Can you work these out from the model? Positions are in its coordinate system, mm. A direction names the side the tool comes from. Coordinates: 2 decimals unless noted, no trailing zeros. Write each loop counter-clockwise with the first axis right and the second up, starting at its lowest first coordinate (ties: lowest second). Pieces come first, ordered by that corner, then holes. Notation, with made-up numbers: (-13, 87.5) - (-6, 87.5) arc R30 cw to (-6, 121.5) - close; hole circle Ø1 at (51.5, 73.5). An arc over 180 degrees is marked (long way). Use one line per item in the form item = value. Start each with the question number.
(1) If I drill on probe 1 along X at (y, z) = (1.7, 10); probe 2 along Z at (x, y) = (-17.5, 3); probe 3 along Z at (x, y) = (17.5, 1.85), over which ranges is the centre line in solid material (lowest first)? Write a range as from..to.
(2) If we section it at C-C on y = 3.1: Please give me the cut outline in (x, z).
(3) On a 3-axis mill with a long thin cutter (end or side, diameter ignored), from which of +Z, -Z, +X, -X, +Y, -Y can I reach the whole of each face in a straight line? I mean faces 1 (the face through (-50, 2, -9)), 2 (the face through (-25, 2, 2)). Say none if no direction works.
(4) Thinking about a two-plate mould opening in Z: for faces 3 (the face through (-18.51, 2.53, -11.11)), 4 (the face through (-1, 5, -4)), 5 (the face through (1, 2, -17.5)), which applies, pulls with the +Z half, pulls with the -Z half, needs draft (parallel to the pull), parting line crosses it, or undercut?
(5) If we section it at B-B on x = -7: Please give me the cut outline in (y, z).
(6) For pin 1 Ø2.5 at (x, z) = (17.5, 10) entering from +Y, with a flat end and sliding along its axis, tell me the tip position at first contact or that it passes through.
(7) If we section it at D-D on x = -17.5: Give the number of separate pieces and of enclosed holes in the cut face, then the cut area to 3 significant figures.
(8) If we section it at A-A on z = 10: Please give me the cut outline in (x, y), then the cut area to 3 significant figures.
```python
from build123d import *

# Parameters (mm, degrees)
BOSS_EXTRUDE1_DEPTH            = 5
F_3_0MM_DOWEL_HOLE1_AT_2_COUNT = 2
F_3_0MM_DOWEL_HOLE1_AT_2_PITCH = 40.311288741
M5_CLEARANCE_HOLE1_AT_2_COUNT  = 2
M5_CLEARANCE_HOLE1_AT_2_PITCH  = 40.311288741
CHAMFER1_SIZE                  = 1
CHAMFER2_SIZE                  = 0.2


with BuildPart() as part:
    # Sketch2 → Boss-Extrude1 (new body)
    with BuildSketch(Plane(origin=(0, 0, 0), x_dir=(1, 0, 0), z_dir=(0, 1, 0))):
        with BuildLine():
            Line((-50, 2), (0, 2))
            ThreePointArc((0, 2), (2, 0), (0, -2))
            Line((0, -2), (-50, -2))
            Line((-50, -2), (-50, -17.5))
            Line((-50, -17.5), (50, -17.5))
            Line((50, -17.5), (50, 17.5))
            Line((50, 17.5), (-50, 17.5))
            Line((-50, 17.5), (-50, 2))
        make_face()
    extrude(amount=BOSS_EXTRUDE1_DEPTH)

    # Sketch4 → Ø3.0mm Dowel Hole1 (revolve, cut)
    with BuildSketch(Plane(origin=(-17.5, 5, -10), x_dir=(0, 0, 1), z_dir=(1, 0, 0))):
        Polygon((0, 0), (0, 5), (1.75, 5), (1.5, 4.75), (1.5, 0.25), (1.75, 0), align=None)
    f_3_0mm_dowel_hole1 = revolve(axis=Axis((-17.5, 11.35, -10), (0, -1, 0)), mode=Mode.SUBTRACT)

    # Ø3.0mm Dowel Hole1 at 2: Ø3.0mm Dowel Hole1 ×2
    with Locations(*[Vector(0.8682431421244593, 0, 0.4961389383568337) * (i * F_3_0MM_DOWEL_HOLE1_AT_2_PITCH) for i in range(1, F_3_0MM_DOWEL_HOLE1_AT_2_COUNT)]):
        add(f_3_0mm_dowel_hole1, mode=Mode.SUBTRACT)

    # Sketch6 → M5 Clearance Hole1 (revolve, cut)
    with BuildSketch(Plane(origin=(-17.5, 5, 10), x_dir=(0, 0, 1), z_dir=(1, 0, 0))):
        Polygon((0, 0), (0, 5), (3, 5), (2.75, 4.75), (2.75, 0.25), (3, 0), align=None)
    m5_clearance_hole1 = revolve(axis=Axis((-17.5, 11.35, 10), (0, -1, 0)), mode=Mode.SUBTRACT)

    # M5 Clearance Hole1 at 2: M5 Clearance Hole1 ×2
    with Locations(*[Vector(0.8682431421244592, 0, -0.4961389383568339) * (i * M5_CLEARANCE_HOLE1_AT_2_PITCH) for i in range(1, M5_CLEARANCE_HOLE1_AT_2_COUNT)]):
        add(m5_clearance_hole1, mode=Mode.SUBTRACT)

    # Chamfer1
    chamfer1_edges = [part.edges().sort_by_distance(p)[0] for p in [
        (50, 2.5, 17.5),
        (-50, 2.5, 17.5),
        (-50, 2.5, -17.5),
        (50, 2.5, -17.5),
    ]]
    chamfer(chamfer1_edges, length=CHAMFER1_SIZE)

    # Chamfer2
    chamfer2_edges = [part.edges().sort_by_distance(p)[0] for p in [
        (-25, 0, -2),
        (-25, 5, -2),
        (2, 5, 0),
        (-25, 5, 2),
        (-50, 5, 9.25),
        (0, 0, -17.5),
        (0, 5, -17.5),
        (50, 0, 0),
        (0, 0, 17.5),
        (-50, 0, -9.25),
        (-49.5, 0, -17),
        (-49.5, 0, 17),
        (49.5, 0, 17),
        (49.5, 0, -17),
        (50, 5, 0),
        (-50, 5, -9.25),
        (0, 5, 17.5),
        (-49.5, 5, -17),
        (-49.5, 5, 17),
        (49.5, 5, 17),
        (49.5, 5, -17),
        (-50, 0, 9.25),
        (-25, 0, 2),
        (2, 0, 0),
    ]]
    chamfer(chamfer2_edges, length=CHAMFER2_SIZE)


solid = part.part
```
Reported:
q1.probe_1 = -50..-20.25, -14.75..16, 19..50
q1.probe_2 = -17.5..-11.5, -8.5..-2, 2..7.25, 12.75..17.5
q1.probe_3 = -17.5..-12.75, -7.25..8.5, 11.5..17.5
q2.outline = (-50, -16.5) - (-49, -17.5) - (49, -17.5) - (50, -16.5) - (50, 16.5) - (49, 17.5) - (-49, 17.5) - (-50, 16.5) - (-50, 2) - (0, 2) arc R2 cw to (0, -2) - (-50, -2) - close; hole circle Ø5.5 at (-17.5, 10); hole circle Ø3 at (-17.5, -10); hole circle Ø5.5 at (17.5, -10); hole circle Ø3 at (17.5, 10)
q3.face_1 = +Z, -Z, -X, +Y, -Y
q3.face_2 = -X, +Y, -Y
q4.face_3 = undercut
q4.face_4 = needs draft
q4.face_5 = pulls with the -Z half
q5.outline = (0, -17.3) - (0.2, -17.5) - (4.8, -17.5) - (5, -17.3) - (5, -2.2) - (4.8, -2) - (0.2, -2) - (0, -2.2) - close; (0, 2.2) - (0.2, 2) - (4.8, 2) - (5, 2.2) - (5, 17.3) - (4.8, 17.5) - (0.2, 17.5) - (0, 17.3) - close
q6.pin_1 = through
q7.separate_pieces = 4
q7.enclosed_holes = 0
q7.area = 112 mm2
q8.outline = (-50, 0.2) - (-49.8, 0) - (-20.5, 0) - (-20.25, 0.25) - (-20.25, 4.75) - (-20.5, 5) - (-49.8, 5) - (-50, 4.8) - close; (-14.75, 0.25) - (-14.5, 0) - (15.75, 0) - (16, 0.25) - (16, 4.75) - (15.75, 5) - (-14.5, 5) - (-14.75, 4.75) - close; (19, 0.25) - (19.25, 0) - (49.8, 0) - (50, 0.2) - (50, 4.8) - (49.8, 5) - (19.25, 5) - (19, 4.75) - close
q8.area = 457 mm2
